Autodesk Inventor part; units mm, degrees
ref_plane "YZ Plane" through (0, 0, 0) normal (1, 0, 0) x (0, 1, 0)
ref_plane "XZ Plane" through (0, 0, 0) normal (0, 1, 0) x (-1, 0, 0)
ref_plane "XY Plane" through (0, 0, 0) normal (0, 0, 1) x (1, 0, 0)
sketch "Sketch1" plane through (0, 0, 0) normal (0, 1, 0) x (-1, 0, 0)
  line L0 (0, 0) -> (22, 0)
  line L1 (22, 0) -> (22, -11.5)
  line L2 (22, -11.5) -> (0, -11.5)
  line L3 (0, -11.5) -> (0, 0)
  dimension "d0" = 22
  dimension "d1" = 11.5
extrude "Extrusion1" add sketch "Sketch1" along normal blind 22.5
fillet "Fillet1" radius 1 4 edges at (-22, 11.25, -11.5) (-22, 11.25, 0) (0, 11.25, 0) (0, 11.25, -11.5)
sketch "Sketch2" plane through (-22, 0, -10.5) normal (-1, 0, 0) x (0, 0, 1)
  point P0 (10.5, 0)
sketch "Sketch3" plane through (0, 22.5, 0) normal (0, 1, 0) x (1, 0, 0)
  circle A0 centre (-16, 5.75) radius 3.5
  line L0 (0, 1) -> (0, 10.5)
  line L1 (-21, 0) -> (-1, 0)
  point P0 (0, 0)
  dimension "d5" = 7
  dimension "d6" = 16
  dimension "d7" = 5.75
extrude "Extrusion2" add sketch "Sketch3" along normal blind 3
properties part number "SG-90-servo-motor"
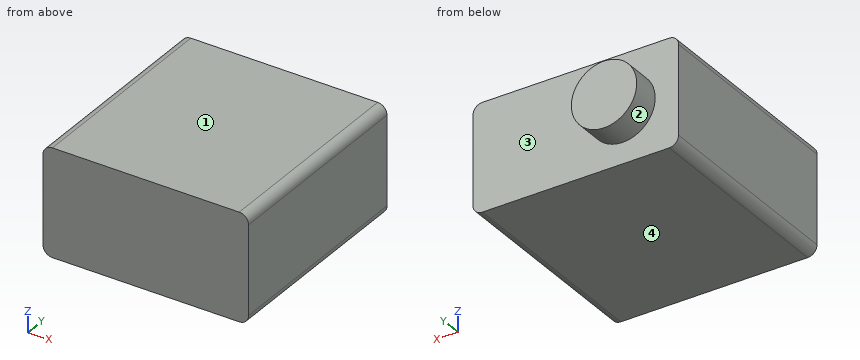
Can you work these out from the model? Positions are in its coordinate system, mm. Face numbers are marked on the shaded views. Give positions to 0.01 mm unless a question says otherwise; leave off trailing zeros. Loops run counter-clockwise (first coordinate to the right, second up) from the corner with the lowest first, then second, coordinate; pieces in that order, holes last. Notation, with made-up numbers: M 22,-23.75 L 53,-23.75 A25 ccw 53,-10.75 Z; hole C 45,46 d1. An arc over 180 degrees is marked long. One line per item, written item: value.
(1) I need wall thicknesses on line 1 (Y direction, x = -7.5, z = -8.25); line 2 (X direction, y = 23, z = -2.75); line 3 (X direction, y = 22.25, z = -0.5). Which ranges of each line are inside material? Lowest first, please.
Returned:
line 1: 0 to 22.5
line 2: -17.8 to -14.2
line 3: -21.87 to -0.13
(2) We'd pull the mould along Z, two halves only. Please class the marked faces 1, 2, 3 and 4: released by +Z, released by -Z, zero draft, split by the parting line, or undercut.
Returned:
face 1: released by +Z
face 2: split by the parting line
face 3: zero draft
face 4: released by -Z
(3) Suppose I cut it at C-C on y = 23.5. List the corners of the cut face in (x, z) for me, plus the area to 3 significant figures.
Returned:
outline: C -16,-5.75 d7
area: 38.5 mm^2
(4) Suppose I cut it at D-D on x = -4.5. List the corners of the cut face in (y, z) for me, plus the area to 3 significant figures.
Returned:
outline: M 0,-11.5 L 22.5,-11.5 L 22.5,0 L 0,0 Z
area: 259 mm^2
(5) Suppose I cut it at A-A on z = -5.75. List the corners of the cut face in (x, y) for me, plus the area to 3 significant figures.
Returned:
outline: M -22,0 L 0,0 L 0,22.5 L -12.5,22.5 L -12.5,25.5 L -19.5,25.5 L -19.5,22.5 L -22,22.5 Z
area: 516 mm^2
(6) Will these pins go through, and if not, where does the flat tip stop? pin 1 (4 mm diameter, centred on x = -19.5, y = 17, fed in from +Z); pin 2 (3 mm diameter, centred on x = -7, z = -5.5, fed in from +Y).
Returned:
pin 1: z = 0
pin 2: y = 22.5
(7) Suppose I cut it at B-B on x = -16. List the corners of the cut face in (y, z) for me, plus the area to 3 significant figures.
Returned:
outline: M 0,-11.5 L 22.5,-11.5 L 22.5,-9.25 L 25.5,-9.25 L 25.5,-2.25 L 22.5,-2.25 L 22.5,0 L 0,0 Z
area: 280 mm^2
